The model under review builds one solid part; all positions refer to its coordinate system, in mm. Coordinates: 2 decimals unless noted, no trailing zeros. Write each loop counter-clockwise with the first axis right and the second up, starting at its lowest first coordinate (ties: lowest second). Pieces come first, ordered by that corner, then holes.
1) For line 1 (X direction, y = 366, z = 1.9); line 2 (Y direction, x = 7, z = 0.8); line 3 (Y direction, x = 101, z = 1.05), list the stretches that pass through material, from the lowest coordinate up.
2) Add section A-A, the plane y = 374.5. State the section outline as (x, z) points.
3) For P1, Ø0.9, axis at y = 443, z = 1, coming from the +X side; P2, Ø0.9, axis at x = 5, z = 1, coming from the +Y side; P3, Ø1.5, axis at y = 1.5, z = 2, coming from the +X side, all flat-tipped, find the tip position at first contact; note any pin that passes through.
Autodesk Inventor part; units mm, degrees
ref_plane "YZ Plane" through (0, 0, 0) normal (1, 0, 0) x (0, 1, 0)
ref_plane "XZ Plane" through (0, 0, 0) normal (0, 1, 0) x (-1, 0, 0)
ref_plane "XY Plane" through (0, 0, 0) normal (0, 0, 1) x (1, 0, 0)
sketch "Sketch1" plane through (0, 0, 0) normal (0, 0, 1) x (1, 0, 0)
  line L0 (0, 0) -> (0, 442)
  line L1 (0, 442) -> (110, 442)
  line L2 (110, 442) -> (110, 0)
  line L3 (110, 0) -> (0, 0)
  line L4 (10, 0) -> (10, 3)
  line L5 (10, 3) -> (0, 3)
  line L6 (100, 0) -> (100, 3)
  line L7 (100, 3) -> (110, 3)
  dimension "d0" = 442
  dimension "d1" = 110
  dimension "d4" = 3
  dimension "d5" = 90
  dimension "d6" = 10
extrude "Extrusion1" add sketch "Sketch1" along normal blind 3 contours L0 L1 L2 L7 L6 L3 L4 L5
sketch "Sketch4" plane through (0, 3, 0) normal (-1, 0, 0) x (0, 0, 1)
  line L0 (3, 439) -> (3, 0)
  line L1 (3, 10) -> (0, 10)
  line L2 (0, 0) -> (3, 0)
  line L3 (0, 439) -> (0, 0)
  line L4 (0, 343) -> (3.087, 343)
  line L5 (0, 439) -> (3, 439)
  point P0 (0, -3)
  point P1 (3, 343)
  dimension "d7" = 10
  dimension "d11" = 333
extrude "Extrusion2" cut sketch "Sketch4" against normal blind 3 contours L0 L2 L3 L1 | L4 L3 L5 L0
sketch "Sketch5" plane through (110, 442, 3) normal (0, 1, 0) x (1, 0, 0)
  line L0 (-10, 3) -> (0, 3)
  line L1 (-5, 3) -> (-5, 0)
  line L2 (-10, 0) -> (0, 0)
  line L3 (-100, 3) -> (-10, 3)
  line L4 (-100, 3) -> (-100, 0)
  line L5 (-100, 0) -> (-10, 0)
  line L6 (-110, 0) -> (-110, 3)
  dimension "d12" = 10
extrude "Extrusion3" add sketch "Sketch5" along normal blind 3
properties part number "lifting cover" material "PMMA Plastic"
Geometry results:
1. line 1: x = 3 to 110
1. line 2: y = 3 to 442
1. line 3: y = 3 to 445
2. outline: (3, 0) - (110, 0) - (110, 3) - (3, 3) - close
3. P1: stops at x = 105
3. P2: stops at y = 442
3. P3: stops at x = 100
